```python
from build123d import *

# Parameters (mm, degrees)
F0_R     = 6
F0_R_2   = 1.5
F1_DEPTH = 2
F2_SIZE  = 1.5


with BuildPart() as f1:
    # F0 (on Front) → F1 (new body)
    with BuildSketch(Plane.XZ):
        Circle(F0_R)
        Circle(F0_R_2, mode=Mode.SUBTRACT)
    extrude(amount=F1_DEPTH)

    # F2
    f2_edges = [f1.edges().sort_by_distance(p)[0] for p in [
        (-6, 0, 0),
    ]]
    chamfer(f2_edges, length=F2_SIZE)

    # F3: F1 across plane


with BuildPart() as f1_1:
    add(f1.part)
    add(f1.part.mirror(Plane.XZ))


solid = f1_1.part
```
Design review of the part built by this model. Coordinates are the model's own, in mm. Give positions to 0.01 mm unless a question says otherwise; leave off trailing zeros. Write each loop counter-clockwise with the first axis right and the second up, starting at its lowest first coordinate (ties: lowest second). Pieces come first, ordered by that corner, then holes. Notation, with made-up numbers: (74, -11.5) -> (108, -11.5) arc R18 cw to (108, 12.5) -> close; hole circle Ø7 at (-37, -19.5). An arc over 180 degrees is marked (long way). Answer in a Markdown table with one row per item.
(1) Consider section B-B (x = 0). State the section outline as (y, z) points.
Results:
| item | result |
|---|---|
| outline | (-2, -6) -> (-1.5, -6) -> (0, -4.5) -> (1.5, -6) -> (2, -6) -> (2, -1.5) -> (-2, -1.5) -> close; (-2, 1.5) -> (2, 1.5) -> (2, 6) -> (1.5, 6) -> (0, 4.5) -> (-1.5, 6) -> (-2, 6) -> close |
(2) Clearance check with flat-ended pins moving along their axes: pin 1 (2.5 mm diameter, centred on x = 0, z = 0, fed in from -Y); pin 2 (2 mm diameter, centred on x = 4.5, y = -0.5, fed in from +Z). State where each tip first meets the part, or that it passes through.
Results:
| item | result |
|---|---|
| pin 1 | through |
| pin 2 | z = 4.3 |
(3) Consider section C-C (y = -0.4). State the section outline as (x, z) points.
Results:
| item | result |
|---|---|
| outline | circle Ø9.8 at (0, 0); hole circle Ø3 at (0, 0) |
(4) Consider section A-A (z = 0). State the section outline as (x, y) points, then the cut area to 3 significant figures.
Results:
| item | result |
|---|---|
| outline | (-6, -2) -> (-1.5, -2) -> (-1.5, 2) -> (-6, 2) -> (-6, 1.5) -> (-4.5, 0) -> (-6, -1.5) -> close; (1.5, -2) -> (6, -2) -> (6, -1.5) -> (4.5, 0) -> (6, 1.5) -> (6, 2) -> (1.5, 2) -> close |
| area | 31.5 mm2 |
(5) Consider section D-D (y = 1.3). State the section outline as (x, z) points, then the cut area to 3 significant figures.
Results:
| item | result |
|---|---|
| outline | circle Ø11.6 at (0, 0); hole circle Ø3 at (0, 0) |
| area | 98.6 mm2 |
(6) To check wall thickness, follow probe 1 along Z at (x, y) = (-0.5, 1); probe 2 along X at (y, z) = (-0.5, -0.5); probe 3 along Z at (x, y) = (0, -0.95). State the ranges of each line that lie inside material, in increasing order.
Results:
| item | result |
|---|---|
| probe 1 | -5.48 to -1.41, 1.41 to 5.48 |
| probe 2 | -4.97 to -1.41, 1.41 to 4.97 |
| probe 3 | -5.45 to -1.5, 1.5 to 5.45 |
